```python
from build123d import *

# Parameters (mm, degrees)
F1_DEPTH = 130
F2_R     = 2.65
F2_R_2   = 13
F2_R_3   = 1.75
F3_DEPTH = 80
F2_R_4   = 19.5
F4_DEPTH = 53
F5_R     = 10
F6_R     = 5
F7_SIZE  = 2
F8_R     = 2
F9_DEPTH = 15


# Not quite as in the source:
# - a feature names something its author has since deleted; it is built from what else it names


with BuildPart() as f1:
    # F0 (on Top) → F1 (new body)
    with BuildSketch(Plane.XY):
        Polygon((35, 90), (-30, 90), (-30, 40), (0, 40), (0, 0), (5, 0), (5, 40), (30, 40), (30, 0), (35, 0), align=None)
    extrude(amount=F1_DEPTH)

    # F2 (on face) → F3 (cut)
    with BuildSketch(Plane.YZ.offset(35)):
        with Locations((10, 120)):
            Circle(F2_R)
        with Locations((10, 10)):
            Circle(F2_R)
        with BuildLine():
            ThreePointArc((10, 35), (11.4644660941, 31.4644660941), (15, 30))
            Line((15, 30), (35, 30))
            ThreePointArc((35, 30), (38.5355339059, 31.4644660941), (40, 35))
            Line((40, 35), (40, 95))
            ThreePointArc((40, 95), (38.5355339059, 98.5355339059), (35, 100))
            Line((35, 100), (15, 100))
            ThreePointArc((15, 100), (11.4644660941, 98.5355339059), (10, 95))
            Line((10, 95), (10, 35))
        make_face()
        with Locations((65, 65)):
            Circle(F2_R_2)
        with Locations((65, 49.5)):
            Circle(F2_R_3)
        with Locations((51.5766062413, 57.25)):
            Circle(F2_R_3)
        with Locations((51.5766062413, 72.75)):
            Circle(F2_R_3)
        with Locations((65, 80.5)):
            Circle(F2_R_3)
        with Locations((78.4233937587, 72.75)):
            Circle(F2_R_3)
        with Locations((78.4233937587, 57.25)):
            Circle(F2_R_3)
        with BuildLine():
            Line((50, 26.5), (50, 7.5))
            ThreePointArc((50, 7.5), (50.1464466094, 7.1464466094), (50.5, 7))
            Line((50.5, 7), (69.5, 7))
            ThreePointArc((69.5, 7), (69.8535533906, 7.1464466094), (70, 7.5))
            Line((70, 7.5), (70, 26.5))
            ThreePointArc((70, 26.5), (69.8535533906, 26.8535533906), (69.5, 27))
            Line((69.5, 27), (50.5, 27))
            ThreePointArc((50.5, 27), (50.1464466094, 26.8535533906), (50, 26.5))
        make_face()
        with BuildLine():
            ThreePointArc((50, 103.5), (50.1464466094, 103.1464466094), (50.5, 103))
            Line((50.5, 103), (69.5, 103))
            ThreePointArc((69.5, 103), (69.8535533906, 103.1464466094), (70, 103.5))
            Line((70, 103.5), (70, 122.5))
            ThreePointArc((70, 122.5), (69.8535533906, 122.8535533906), (69.5, 123))
            Line((69.5, 123), (50.5, 123))
            ThreePointArc((50.5, 123), (50.1464466094, 122.8535533906), (50, 122.5))
            Line((50, 122.5), (50, 103.5))
        make_face()
    extrude(amount=-F3_DEPTH, mode=Mode.SUBTRACT)

    # F2 (on face) → F4 (cut)
    with BuildSketch(Plane.YZ.offset(35)):
        with Locations((65, 65)):
            Circle(F2_R_4)
        with Locations((51.5766062413, 57.25)):
            Circle(F2_R_3, mode=Mode.SUBTRACT)
        with Locations((65, 49.5)):
            Circle(F2_R_3, mode=Mode.SUBTRACT)
        with Locations((78.4233937587, 57.25)):
            Circle(F2_R_3, mode=Mode.SUBTRACT)
        with Locations((51.5766062413, 72.75)):
            Circle(F2_R_3, mode=Mode.SUBTRACT)
        with Locations((65, 65)):
            Circle(F2_R_2, mode=Mode.SUBTRACT)
        with Locations((65, 80.5)):
            Circle(F2_R_3, mode=Mode.SUBTRACT)
        with Locations((78.4233937587, 72.75)):
            Circle(F2_R_3, mode=Mode.SUBTRACT)
    extrude(amount=-F4_DEPTH, mode=Mode.SUBTRACT)

    # F5
    f5_edges = [f1.edges().sort_by_distance(p)[0] for p in [
        (32.5, 0, 130),
        (2.5, 0, 130),
        (32.5, 0, 0),
        (2.5, 0, 0),
        (0, 40, 112.5),
        (0, 40, 17.5),
    ]]
    fillet(f5_edges, radius=F5_R)

    # F6
    f6_edges = [f1.edges().sort_by_distance(p)[0] for p in [
        (5, 40, 112.5),
        (5, 40, 17.5),
        (30, 40, 112.5),
        (30, 40, 17.5),
    ]]
    fillet(f6_edges, radius=F6_R)

    # F7
    f7_edges = [f1.edges().sort_by_distance(p)[0] for p in [
        (-30, 60, 123),
        (-30, 60, 27),
    ]]
    chamfer(f7_edges, length=F7_SIZE)

    # F8 (on face) → F9 (cut)
    with BuildSketch(Plane(origin=(0, 90, 0), x_dir=(-1, 0, 0), z_dir=(0, 1, 0))):
        with Locations((21, 10)):
            Circle(F8_R)
        with Locations((1, 10)):
            Circle(F8_R)
        with Locations((-19, 10)):
            Circle(F8_R)
        with Locations((1, 35)):
            Circle(F8_R)
        with Locations((-19, 35)):
            Circle(F8_R)
        with Locations((21, 35)):
            Circle(F8_R)
        with Locations((21, 95)):
            Circle(F8_R)
        with Locations((1, 95)):
            Circle(F8_R)
        with Locations((-19, 95)):
            Circle(F8_R)
        with Locations((-19, 120)):
            Circle(F8_R)
        with Locations((1, 120)):
            Circle(F8_R)
        with Locations((21, 120)):
            Circle(F8_R)
    extrude(amount=-F9_DEPTH, mode=Mode.SUBTRACT)


solid = f1.part
```
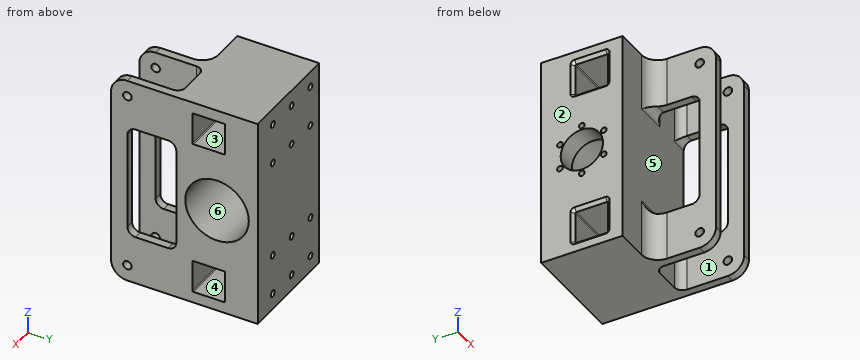
Part model, mm, in its own coordinate system. Face numbers are marked on the shaded views. A direction names the side the tool comes from. Round coordinates to 2 decimals unless told otherwise and drop trailing zeros. Loops run counter-clockwise (first coordinate to the right, second up) from the corner with the lowest first, then second, coordinate; pieces in that order, holes last.
1. Drill centre lines: line 1 along Z through (x, y) = (13, 65); line 2 along Y through (x, z) = (-25.5, 65.5); line 3 along Z through (x, y) = (-21, 82). Where is each one in solid material? Low to high.
Solutions:
line 1: z = 0 to 7, 27 to 45.5, 84.5 to 103, 123 to 130
line 2: y = 40 to 52.01, 77.99 to 90
line 3: z = 0 to 8, 12 to 33, 37 to 93, 97 to 118, 122 to 130
2. Two-plate mould, pull along X, no slides. Class the marked faces 1, 2 and 3: pulls with the +X half, pulls with the -X half, needs draft (parallel to the pull), parting line crosses it, or undercut.
Solutions:
face 1: undercut
face 2: pulls with the -X half
face 3: needs draft
3. Slice it at D-D (z = 115.5). Give the cut face in (x, y).
Solutions:
outline: (-30, 40) - (-10, 40) arc R10 cw to (0, 30) - (0, 0) - (5, 0) - (5, 35) arc R5 cw to (10, 40) - (25, 40) arc R5 cw to (30, 35) - (30, 0) - (35, 0) - (35, 50) - (-28, 50) - (-30, 48) - close; (-30, 72) - (-28, 70) - (35, 70) - (35, 90) - (-30, 90) - close
4. Flat gauge pins, fed straight in: pin 1 (4 mm diameter, centred on y = 78.42, z = 57.25, fed in from +X); pin 2 (3 mm diameter, centred on x = -21, z = 120, fed in from -Y); pin 3 (2 mm diameter, centred on x = 7, z = 13.5, fed in from -Y). Where does each tip first touch, or does it go through?
Solutions:
pin 1: stops at x = -18
pin 2: stops at y = 40
pin 3: stops at y = 38
5. Slice it at A-A (z = 65). Give the cut face in (x, y).
Solutions:
outline: (-30, 40) - (35, 40) - (35, 45.5) - (-18, 45.5) - (-18, 52) - (-30, 52) - close; (-30, 78) - (-18, 78) - (-18, 84.5) - (35, 84.5) - (35, 90) - (-30, 90) - close; (0, 0) - (5, 0) - (5, 10) - (0, 10) - close; (30, 0) - (35, 0) - (35, 10) - (30, 10) - close
6. Slice it at B-B (y = 27). Give the cut face in (x, z).
Solutions:
outline: (0, 0) - (5, 0) - (5, 30) - (0, 30) - close; (0, 100) - (5, 100) - (5, 130) - (0, 130) - close; (30, 0) - (35, 0) - (35, 30) - (30, 30) - close; (30, 100) - (35, 100) - (35, 130) - (30, 130) - close
7. 3-axis set-ups, long thin cutter, end or side, ignore diameter. For the marked faces 4, 5 and 6: which of +Z, -Z, +X, -X, +Y, -Y reach the whole face in a straight line?
Solutions:
face 4: +X, -X
face 5: none
face 6: +X
8. Slice it at C-C (x = 12.5). Give the cut face in (y, z), and give its area (3 significant figures).
Solutions:
outline: (40, 0) - (90, 0) - (90, 130) - (40, 130) - close; hole circle Ø39 at (65, 65); hole (50, 7.5) arc R0.5 ccw to (50.5, 7) - (69.5, 7) arc R0.5 ccw to (70, 7.5) - (70, 26.5) arc R0.5 ccw to (69.5, 27) - (50.5, 27) arc R0.5 ccw to (50, 26.5) - close; hole (50, 103.5) arc R0.5 ccw to (50.5, 103) - (69.5, 103) arc R0.5 ccw to (70, 103.5) - (70, 122.5) arc R0.5 ccw to (69.5, 123) - (50.5, 123) arc R0.5 ccw to (50, 122.5) - close
area: 4,510 mm2
